Here's how the part is built. I have some questions about the finished solid (model axes, mm). A direction names the side the tool comes from. Give positions to 0.01 mm unless a question says otherwise; leave off trailing zeros. Loops run counter-clockwise (first coordinate to the right, second up) from the corner with the lowest first, then second, coordinate; pieces in that order, holes last. Notation, with made-up numbers: (-6, 40) - (17, 40) arc R17 ccw to (17, 52) - close; hole circle Ø6 at (43.5, -35.75). An arc over 180 degrees is marked (long way). Use a Markdown table: item, result.
from build123d import *

# Parameters (mm, degrees)
F0_R     = 1
F0_R_2   = 0.8289430236
F1_DEPTH = 3
F0_W     = 10
F0_H     = 2.9
F2_DEPTH = 10
F3_R     = 4.99999
F5_R     = 0.5
F4_R     = 1.55
F6_DEPTH = 8.9


# Not quite as in the source:
# - a fillet or chamfer is up to 0.001 mm smaller than in the source, because OpenCascade refuses the exact size


with BuildPart() as f1:
    # F0 (on Top) → F1 (new body)
    with BuildSketch(Plane.XY):
        with BuildLine():
            ThreePointArc((11.75, 10.5), (11.1642135624, 11.9142135624), (9.75, 12.5))
            Line((9.75, 12.5), (-9.75, 12.5))
            ThreePointArc((-9.75, 12.5), (-11.1642135624, 11.9142135624), (-11.75, 10.5))
            Line((-11.75, 10.5), (-11.75, 8.5))
            ThreePointArc((-11.75, 8.5), (-11.1642135624, 7.0857864376), (-9.75, 6.5))
            Line((-9.75, 6.5), (6.25, 6.5))
            ThreePointArc((6.25, 6.5), (7.6642135624, 5.9142135624), (8.25, 4.5))
            Line((8.25, 4.5), (8.25, -4.5))
            ThreePointArc((8.25, -4.5), (7.6642135624, -5.9142135624), (6.25, -6.5))
            Line((6.25, -6.5), (-9.75, -6.5))
            ThreePointArc((-9.75, -6.5), (-11.1642135624, -7.0857864376), (-11.75, -8.5))
            Line((-11.75, -8.5), (-11.75, -10.5))
            ThreePointArc((-11.75, -10.5), (-11.1642135624, -11.9142135624), (-9.75, -12.5))
            Line((-9.75, -12.5), (9.75, -12.5))
            ThreePointArc((9.75, -12.5), (11.1642135624, -11.9142135624), (11.75, -10.5))
            Line((11.75, -10.5), (11.75, -4.45))
            Line((11.75, -4.45), (11.75, -1.55))
            Line((11.75, -1.55), (11.75, 1.55))
            Line((11.75, 1.55), (11.75, 4.45))
            Line((11.75, 4.45), (11.75, 10.5))
        make_face()
        with Locations((-9.75, -10.5)):
            Circle(F0_R, mode=Mode.SUBTRACT)
        with Locations((2.9210569764, -10.6710569764)):
            Circle(F0_R_2, mode=Mode.SUBTRACT)
        with Locations((-9.75, 10.5)):
            Circle(F0_R, mode=Mode.SUBTRACT)
        with Locations((2.75, 10.5)):
            Circle(F0_R, mode=Mode.SUBTRACT)
    extrude(amount=F1_DEPTH)

    # F0 (on Top) → F2 (join)
    with BuildSketch(Plane.XY):
        with Locations((16.75, 3)):
            Rectangle(F0_W, F0_H)
        with Locations((16.75, -3)):
            Rectangle(F0_W, F0_H)
    extrude(amount=F2_DEPTH)

    # F3 (radius 5 in the source; OpenCascade refuses exactly that, so slightly less here)
    f3_edges = [f1.edges().sort_by_distance(p)[0] for p in [
        (11.75, -3, 10),
        (11.75, 3, 10),
        (21.75, 3, 10),
        (21.75, -3, 10),
        (21.75, 3, 0),
        (21.75, -3, 0),
    ]]
    fillet(f3_edges, radius=F3_R)

    # F5
    f5_edges = [f1.edges().sort_by_distance(p)[0] for p in [
        (-1.75, 6.5, 3),
        (11.75, 7.475, 3),
        (11.75, 0, 3),
        (11.75, -7.475, 3),
        (0, -12.5, 0),
        (11.75, 0, 0),
    ]]
    fillet(f5_edges, radius=F5_R)

    # F4 (on face) → F6 (cut)
    with BuildSketch(Plane.XZ.offset(4.45)):
        with Locations((16.75, 5)):
            Circle(F4_R)
    extrude(amount=-F6_DEPTH, mode=Mode.SUBTRACT)


solid = f1.part
(1) Will these pins go through, and if not, where does the flat tip stop? pin 1 (5 mm diameter, centred on x = 19, z = 6, fed in from -Y); pin 2 (5 mm diameter, centred on x = 14.5, z = 6, fed in from +Y); pin 3 (1 mm diameter, centred on y = 3, z = 4, fed in from -X); pin 4 (3 mm diameter, centred on x = 2.75, y = 10.5, fed in from -Z).
A:
| item | result |
|---|---|
| pin 1 | y = -4.45 |
| pin 2 | y = 4.45 |
| pin 3 | x = 11.75 |
| pin 4 | z = 0 |
(2) Suppose I cut it at D-D on y = -0.5. Write out the boundary of the cut face in (x, z).
A:
| item | result |
|---|---|
| outline | (8.25, 0.5) arc R0.5 ccw to (8.75, 0) - (11.25, 0) arc R0.5 ccw to (11.75, 0.5) - (11.75, 2.5) arc R0.5 ccw to (11.25, 3) - (8.75, 3) arc R0.5 ccw to (8.25, 2.5) - close |
(3) We'd pull the mould along Z, two halves only. Please class faces 6 (the face through (-10.487, 11.176, 1.479)), 7 (the face through (3, 8, 3)), 8 (the face through (15.2, -3.02, 5.07)): pulls with the +Z half, pulls with the -Z half, needs draft (parallel to the pull), parting line crosses it, or undercut.
A:
| item | result |
|---|---|
| face 6 | needs draft |
| face 7 | pulls with the +Z half |
| face 8 | undercut |
(4) On a 3-axis mill with a long thin cutter (end or side, diameter ignored), from which of +Z, -Z, +X, -X, +Y, -Y can I reach the whole of each face in a straight line? I mean faces 1 (the face through (-11.18, 7.1, 1.49)), 2 (the face through (11.75, 3, 4)), 3 (the face through (11.75, 7, 1)), 4 (the face through (11.75, -8, 1)), 5 (the face through (11.75, 0, 1)). Say none if no direction works.
A:
| item | result |
|---|---|
| face 1 | +Z, -Z, -X |
| face 2 | +Z, -X, +Y, -Y |
| face 3 | +Z, -Z, +X, +Y |
| face 4 | +Z, -Z, +X, -Y |
| face 5 | +Z, -Z, +X |
(5) If I drill on line 1 (Y direction, x = -9.75, z = 1.45); line 2 (Z direction, x = 16.75, y = 2.4); line 3 (Y direction, x = 14, z = 5), over which ranges is the centre line in solid material (lowest first)?
A:
| item | result |
|---|---|
| line 1 | -12.5 to -11.5, -9.5 to -6.5, 6.5 to 9.5, 11.5 to 12.5 |
| line 2 | 0 to 3.45, 6.55 to 10 |
| line 3 | -4.45 to -1.55, 1.55 to 4.45 |
(6) Suppose I cut it at B-B on z = 9.25. Write out the boundary of the cut face in (x, y).
A:
| item | result |
|---|---|
| outline | (14.12, -4.45) - (19.38, -4.45) - (19.38, -1.55) - (14.12, -1.55) - close; (14.12, 1.55) - (19.38, 1.55) - (19.38, 4.45) - (14.12, 4.45) - close |
(7) Suppose I cut it at C-C on x = 0. Write out the boundary of the cut face in (y, z), plus the area to 3 significant figures.
A:
| item | result |
|---|---|
| outline | (-12.5, 0.5) arc R0.5 ccw to (-12, 0) - (-7, 0) arc R0.5 ccw to (-6.5, 0.5) - (-6.5, 2.5) arc R0.5 ccw to (-7, 3) - (-12, 3) arc R0.5 ccw to (-12.5, 2.5) - close; (6.5, 0.5) arc R0.5 ccw to (7, 0) - (12, 0) arc R0.5 ccw to (12.5, 0.5) - (12.5, 2.5) arc R0.5 ccw to (12, 3) - (7, 3) arc R0.5 ccw to (6.5, 2.5) - close |
| area | 35.6 mm2 |
